Design review of the part shown in the three views and the two pictorial views. Dimensions are in mm from the part's minimum x, y and z. Coordinates: 2 decimals unless noted, no trailing zeros. Write each loop counter-clockwise with the first axis right and the second up, starting at its lowest first coordinate (ties: lowest second). Pieces come first, ordered by that corner, then holes. Notation, with made-up numbers: M 71.5,82 L 101.5,82 A37 ccw 101.5,119 Z; hole C 39,-23.5 d3. An arc over 180 degrees is marked long. One line per question, with ' | ' between items.
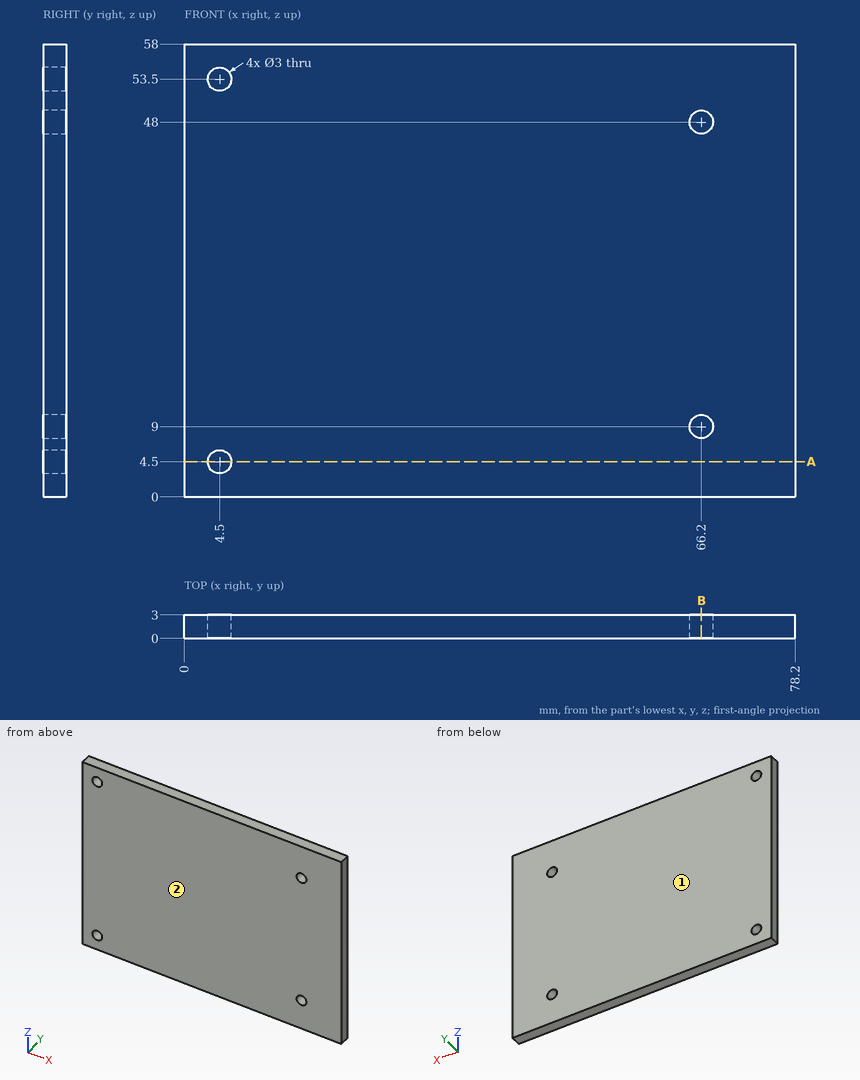
1. Clearance check with a flat-ended pin moving along its axis: P1, Ø5, axis at x = 4.5, z = 53.5, coming from the +Y side. State where the tip first meets the part, or that it passes through.
Computed values:
P1: stops at y = 3
2. For line 1 along X through (y, z) = (1.25, 48); line 2 along X through (y, z) = (1.7, 4.5); line 3 along Z through (x, y) = (67, 1.8), list the stretches that pass through material, from the lowest coordinate up.
Computed values:
line 1: x = 0 to 64.7, 67.7 to 78.2 | line 2: x = 0 to 3, 6 to 78.2 | line 3: z = 0 to 7.73, 10.27 to 46.73, 49.27 to 58
3. Take a section at A-A on z = 4.5. State the section outline as (x, y) points.
Computed values:
outline: M 0,0 L 3,0 L 3,3 L 0,3 Z; M 6,0 L 78.2,0 L 78.2,3 L 6,3 Z
4. Take a section at B-B on x = 66.2. State the section outline as (y, z) points.
Computed values:
outline: M 0,0 L 3,0 L 3,7.5 L 0,7.5 Z; M 0,10.5 L 3,10.5 L 3,46.5 L 0,46.5 Z; M 0,49.5 L 3,49.5 L 3,58 L 0,58 Z
5. Draft analysis for pull direction Y (two halves, no side actions). For the marked faces 1 and 2, state which applies: pulls with the +Y half, pulls with the -Y half, needs draft (parallel to the pull), parting line crosses it, or undercut.
Computed values:
face 1: pulls with the +Y half | face 2: pulls with the -Y half
